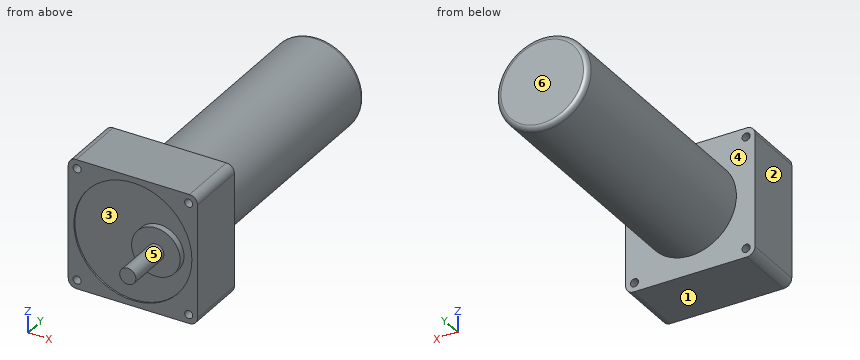
from build123d import *

# Parameters (mm, degrees)
SKETCH1_W           = 80
SKETCH1_H           = 80
BOSS_EXTRUDE1_DEPTH = 38
SKETCH2_R           = 28.5
BOSS_EXTRUDE2_DEPTH = 153
SKETCH3_R           = 36.5
CUT_EXTRUDE1_DEPTH  = 1
SKETCH4_R           = 15
BOSS_EXTRUDE3_DEPTH = 4
SKETCH5_R           = 5
BOSS_EXTRUDE4_DEPTH = 29
FILLET1_R           = 5
SKETCH6_R           = 2.5
CUT_EXTRUDE2_DEPTH  = 38
SKETCH7_R           = 2.5
CUT_EXTRUDE3_DEPTH  = 38
FILLET2_R           = 3


with BuildPart() as part:
    # Sketch1 → Boss-Extrude1 (new body)
    with BuildSketch(Plane(origin=(0, 0, 0), x_dir=(1, 0, 0), z_dir=(0, 1, 0))):
        Rectangle(SKETCH1_W, SKETCH1_H)
    extrude(amount=BOSS_EXTRUDE1_DEPTH)

    # Sketch2 → Boss-Extrude2 (add)
    with BuildSketch(Plane(origin=(0, 38, 0), x_dir=(1, 0, 0), z_dir=(0, 1, 0))):
        Circle(SKETCH2_R)
    extrude(amount=BOSS_EXTRUDE2_DEPTH)

    # Sketch3 → Cut-Extrude1 (cut)
    with BuildSketch(Plane.XZ):
        Circle(SKETCH3_R)
    extrude(amount=-CUT_EXTRUDE1_DEPTH, mode=Mode.SUBTRACT)

    # Sketch4 → Boss-Extrude3 (add)
    with BuildSketch(Plane.XZ.offset(-1)):
        with Locations((16, 0)):
            Circle(SKETCH4_R)
    extrude(amount=BOSS_EXTRUDE3_DEPTH)

    # Sketch5 → Boss-Extrude4 (add)
    with BuildSketch(Plane.XZ.offset(3)):
        with Locations((16, 0)):
            Circle(SKETCH5_R)
    extrude(amount=BOSS_EXTRUDE4_DEPTH)

    # Fillet1
    fillet1_edges = [part.edges().sort_by_distance(p)[0] for p in [
        (40, 19, 40),
        (-40, 19, 40),
        (-40, 19, -40),
        (40, 19, -40),
    ]]
    fillet(fillet1_edges, radius=FILLET1_R)

    # Sketch6 → Cut-Extrude2 (cut)
    with BuildSketch(Plane.XZ):
        with Locations((-34.5, 34.5)):
            Circle(SKETCH6_R)
    extrude(amount=-CUT_EXTRUDE2_DEPTH, mode=Mode.SUBTRACT)

    # Sketch7 → Cut-Extrude3 (cut)
    with BuildSketch(Plane.XZ):
        with Locations((34.5, 34.5)):
            Circle(SKETCH7_R)
        with Locations((34.5, -34.5)):
            Circle(SKETCH7_R)
        with Locations((-34.5, -34.5)):
            Circle(SKETCH7_R)
    extrude(amount=-CUT_EXTRUDE3_DEPTH, mode=Mode.SUBTRACT)

    # Fillet2
    fillet2_edges = [part.edges().sort_by_distance(p)[0] for p in [
        (-28.5, 191, 0),
    ]]
    fillet(fillet2_edges, radius=FILLET2_R)


solid = part.part
Build history of the part. All positions in model axes, mm. Face numbers are marked on the shaded views. A direction names the side the tool comes from. Give positions to 0.01 mm unless a question says otherwise; leave off trailing zeros. Order: outer loops, then holes, each group sorted by start corner. A loop starts at its lowest first (then second) coordinate and runs counter-clockwise, first axis right, second up. Notation, with made-up numbers: M 27.5,38.5 L 42.5,38.5 A19 cw 42.5,66.5 Z; hole C 42,48.25 d4. An arc over 180 degrees is marked long. Use one line per item in the form item = value.
Q1. Wall check: probe 1 along X at (y, z) = (28, 34); probe 2 along Y at (x, z) = (-18, 33). Give the ranges that are in metal, low to high.
Conclusion:
probe_1 = -40 to -36.95, -32.05 to 32.05, 36.95 to 40
probe_2 = 0 to 38
Q2. Slice it at A-A, the plane y = 27.5. Write the cut outline in (x, z).
Conclusion:
outline = M -40,-35 A5 ccw -35,-40 L 35,-40 A5 ccw 40,-35 L 40,35 A5 ccw 35,40 L -35,40 A5 ccw -40,35 Z; hole C -34.5,-34.5 d5; hole C -34.5,34.5 d5; hole C 34.5,-34.5 d5; hole C 34.5,34.5 d5
Q3. Slice it at B-B, the plane z = 0. Write the cut outline in (x, y).
Conclusion:
outline = M -40,0 L -36.5,0 L -36.5,1 L 1,1 L 1,-3 L 11,-3 L 11,-32 L 21,-32 L 21,-3 L 31,-3 L 31,1 L 36.5,1 L 36.5,0 L 40,0 L 40,38 L 28.5,38 L 28.5,188 A3 ccw 25.5,191 L -25.5,191 A3 ccw -28.5,188 L -28.5,38 L -40,38 Z
Q4. Which spindle directions (+Z, -Z, +X, -X, +Y, -Y) get a long thin tool onto all of the face, cutting with end or side? Do the marked faces 4, 5 and 6. Say none if no direction does.
Conclusion:
face_4 = +Y
face_5 = -Y
face_6 = +Z, -Z, +X, -X, +Y
Q5. Pull direction Z, two halves, no side cores. Call the marked faces 1, 2 and 3: released by +Z, released by -Z, zero draft, split by the parting line, or undercut.
Conclusion:
face_1 = released by -Z
face_2 = zero draft
face_3 = undercut
Q6. Pin check, flat tips, straight feed: P1, Ø22, axis at x = -14.5, z = -6.5, coming from the -Y side; P2, Ø6, axis at x = 34.5, z = 34.5, coming from the -Y side; P3, Ø3, axis at x = 34.5, z = -34.5, coming from the -Y side; P4, Ø6, axis at x = -17.5, y = 85.5, coming from the +Z side. Stop position of each tip, or through.
Conclusion:
P1 = 1
P2 = 0
P3 = through
P4 = 24.54
